Design review of the part built by this model. Coordinates are the model's own, in mm. A direction names the side the tool comes from. Coordinates: 2 decimals unless noted, no trailing zeros. Loops run counter-clockwise (first coordinate to the right, second up) from the corner with the lowest first, then second, coordinate; pieces in that order, holes last. Notation, with made-up numbers: (-1.75, 81.25) -> (46.25, 81.25) arc R20 ccw to (46.25, 107.25) -> close; hole circle Ø1 at (-12, 86). An arc over 180 degrees is marked (long way). Use one line per item in the form item = value. Start each with the question number.
1. The part is to be moulded in two halves that separate along X. For faces 1 (the face through (2, -2, -39.37)), 2 (the face through (2.435, 0.767, -26.492)), 3 (the face through (4.609, 7.228, 0.356)), say which applies: released by +X, released by -X, zero draft, split by the parting line, or undercut.
2. For pin 1 (8 mm diameter, centred on x = 6.5, y = -6.5, fed in from +Z); pin 2 (1 mm diameter, centred on x = 1, z = -14, fed in from -Y); pin 3 (1.5 mm diameter, centred on x = 4.5, y = 4.5, fed in from +Z), all flat-tipped, find the tip position at first contact; note any pin that passes through.
3. Wall thickness on line 1 (Y direction, x = 0, z = -28); line 2 (Y direction, x = 0, z = 26); line 3 (Z direction, x = 1.5, y = 6.5): over which ranges is each line inside the solid? List them lowest first. Write a range as from..to.
4. Machinability: for faces 4 (the face through (2, -2, 39.37)), 5 (the face through (-1.38, -6.2, -32.3)), 6 (the face through (-1.38, -6.2, 32.47)), which of the approach directions +Z, -Z, +X, -X, +Y, -Y give a long, thin tool a straight path to every point of the face, cutting with its end or side? Answer none if there is none.
5. Consider section A-A (z = -15). State the section outline as (x, y) points (1 decimal), then the cut area to 3 significant figures.
from build123d import *

# Parameters (mm, degrees)
SKETCH1_R                   = 8.5725
SKETCH1_R_2                 = 6.35
BOSS_EXTRUDE1_DEPTH         = 26.67
SKETCH2_R                   = 6.35
BOSS_EXTRUDE2_DEPTH         = 39.37
CHAMFER1_SIZE               = 1.27
F_1_4_20_TAPPED_HOLE1_D     = 5.1054
F_1_4_20_TAPPED_HOLE1_DEPTH = 25.4
F_1_4_20_TAPPED_HOLE1_TIP   = 1.533816902
F_1_4_20_TAPPED_HOLE2_D     = 5.1054
F_1_4_20_TAPPED_HOLE2_DEPTH = 25.4
F_1_4_20_TAPPED_HOLE2_TIP   = 1.533816902


with BuildPart() as part:
    # Sketch1 → Boss-Extrude1 (new body, symmetric)
    with BuildSketch(Plane.XY):
        Circle(SKETCH1_R)
        Circle(SKETCH1_R_2, mode=Mode.SUBTRACT)
    extrude(amount=BOSS_EXTRUDE1_DEPTH, both=True)

    # Sketch2 → Boss-Extrude2 (add, symmetric)
    with BuildSketch(Plane.XY):
        Circle(SKETCH2_R)
    extrude(amount=BOSS_EXTRUDE2_DEPTH, both=True)

    # Chamfer1
    chamfer1_edges = [part.edges().sort_by_distance(p)[0] for p in [
        (-8.5725, 0, -26.67),
        (-8.5725, 0, 26.67),
        (-6.35, 0, -39.37),
        (-6.35, 0, 39.37),
    ]]
    chamfer(chamfer1_edges, length=CHAMFER1_SIZE)

    # 1/4-20 Tapped Hole1
    with Locations(Plane(origin=(0, 0, -39.37), x_dir=(-1, 0, 0), z_dir=(0, 0, -1))):
        with Locations((0, 0)):
            Hole(F_1_4_20_TAPPED_HOLE1_D / 2, depth=F_1_4_20_TAPPED_HOLE1_DEPTH)
            with Locations((0, 0, -(F_1_4_20_TAPPED_HOLE1_DEPTH + F_1_4_20_TAPPED_HOLE1_TIP / 2))):  # 118° drill point
                Cone(0, F_1_4_20_TAPPED_HOLE1_D / 2, F_1_4_20_TAPPED_HOLE1_TIP, mode=Mode.SUBTRACT)

    # 1/4-20 Tapped Hole2
    with Locations(Plane.XY.offset(39.37)):
        with Locations((0, 0)):
            Hole(F_1_4_20_TAPPED_HOLE2_D / 2, depth=F_1_4_20_TAPPED_HOLE2_DEPTH)
            with Locations((0, 0, -(F_1_4_20_TAPPED_HOLE2_DEPTH + F_1_4_20_TAPPED_HOLE2_TIP / 2))):  # 118° drill point
                Cone(0, F_1_4_20_TAPPED_HOLE2_D / 2, F_1_4_20_TAPPED_HOLE2_TIP, mode=Mode.SUBTRACT)


solid = part.part
Geometry check:
q1.face_1 = zero draft
q1.face_2 = undercut
q1.face_3 = split by the parting line
q2.pin_1 = 39.26
q2.pin_2 = -8.56
q2.pin_3 = 38.84
q3.line_1 = -6.35..-2.55, 2.55..6.35
q3.line_2 = -7.97..-2.55, 2.55..7.97
q3.line_3 = -26.67..26.67
q4.face_4 = +Z, +X, -X, +Y, -Y
q4.face_5 = -Z
q4.face_6 = +Z
q5.outline = circle Ø17.1 at (0, 0); hole circle Ø5.1 at (0, 0)
q5.area = 210 mm²
